from build123d import *

# Parameters (mm, degrees)
EXTRUDE_1_DEPTH      = 30
HOLE_WIZARD_M3_1_D   = 2.5
EXTRUDE_3_DEPTH      = 6
EXTRUDE_3_DEPTH_BACK = 5
SKETCH_4_R           = 1.5


with BuildPart() as part:
    # 草图1 → 凸台-拉伸1 (new body)
    with BuildSketch(Plane(origin=(0, 0, 0), x_dir=(1, 0, 0), z_dir=(0, 1, 0))):
        Polygon((1.5, 2.598076211), (-1.5, 2.598076211), (-3, 0), (-1.5, -2.598076211), (1.5, -2.598076211), (3, 0), align=None)
    extrude(amount=EXTRUDE_1_DEPTH)

    # M3 螺纹孔1 (through all)
    with Locations(Plane(origin=(0, 30, 0), x_dir=(1, 0, 0), z_dir=(0, 1, 0))):
        with Locations((0, 0)):
            Hole(HOLE_WIZARD_M3_1_D / 2)

    # 草图4 → 凸台-拉伸3 (add, two sides: drawn at the far end of the back side and taken through both)
    with BuildSketch(Plane(origin=(0, 30, 0), x_dir=(1, 0, 0), z_dir=(0, 1, 0)).offset(-EXTRUDE_3_DEPTH_BACK)):
        with Locations(Location((0, 0, 0), (0, 0, 270))):
            Circle(SKETCH_4_R)
    extrude(amount=EXTRUDE_3_DEPTH + EXTRUDE_3_DEPTH_BACK)


solid = part.part
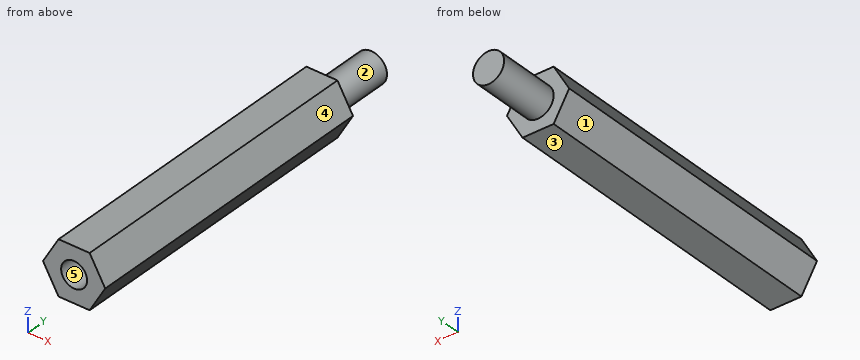
Work out the finished part from the listing and answer in its coordinate system (mm). Face numbers are marked on the shaded views. A direction names the side the tool comes from. Give positions to 0.01 mm unless a question says otherwise; leave off trailing zeros. Order: outer loops, then holes, each group sorted by start corner. A loop starts at its lowest first (then second) coordinate and runs counter-clockwise, first axis right, second up. Notation, with made-up numbers: (89, 37) - (101, 37) arc R13 cw to (101, 43) - close; hole circle Ø1 at (51, 23.5). An arc over 180 degrees is marked (long way). Answer as CSV lines item,"result". Start each with the question number.
Q1. The mould has two halves that part along X. Classify the marked faces 3, 4 and 5: +X half, -X half, draft (parallel to the pull), parting line (faces both ways), or undercut.
Q2. Find the intervals of material crossed by L1, parallel to Z at x = 0, y = 12.5; L2, parallel to Y at x = -2, z = -1.55; L3, parallel to X at y = 4, z = 0.8, in increasing order. Write a range as [from, to].
Q3. For the marked faces 1 and 2, determine the directions among +Z, -Z, +X, -X, +Y, -Y from which every point of the face is accessible in a straight line to the end or side of a thin tool.
Q4. The part is cut by section D-D (z = -1.9). Write down the section's boundary in (x, y).
Q5. The part is cut by section B-B (x = 0). Write down the section's boundary in (y, z), then the cut area to 3 significant figures.
Q6. The part is cut by section C-C (y = 28). Write down the section's boundary in (x, z).
Q7. Given pin 1 Ø0.8 at (x, z) = (0, -0.5) entering from -Y; pin 2 Ø3 at (x, z) = (0, 0) entering from -Y, each flat-ended and moving along its own axis, determine where each tip first touches the part or whether it passes through.
Q8. The part is cut by section A-A (y = 21). Write down the section's boundary in (x, z).
Check result:
1,face 3,"draft"
1,face 4,"+X half"
1,face 5,"undercut"
2,L1,"z = [-2.6, -1.25], [1.25, 2.6]"
2,L2,"y = [0, 30]"
2,L3,"x = [-2.54, -0.96], [0.96, 2.54]"
3,face 1,"-Z, -X, +Y, -Y"
3,face 2,"+Y"
4,outline,"(-1.9, 0) - (1.9, 0) - (1.9, 30) - (-1.9, 30) - close"
5,outline,"(0, -2.6) - (30, -2.6) - (30, -1.5) - (36, -1.5) - (36, 1.5) - (30, 1.5) - (30, 2.6) - (0, 2.6) - (0, 1.25) - (25, 1.25) - (25, -1.25) - (0, -1.25) - close"
5,area,"111 mm²"
6,outline,"(-3, 0) - (-1.5, -2.6) - (1.5, -2.6) - (3, 0) - (1.5, 2.6) - (-1.5, 2.6) - close"
7,pin 1,"stops at y = 25"
7,pin 2,"stops at y = 0"
8,outline,"(-3, 0) - (-1.5, -2.6) - (1.5, -2.6) - (3, 0) - (1.5, 2.6) - (-1.5, 2.6) - close; hole circle Ø2.5 at (0, 0)"
